Geometry: final body of the model. Coordinates: model frame, mm. Coordinates: 2 decimals unless noted, no trailing zeros. Order: outer loops, then holes, each group sorted by start corner. A loop starts at its lowest first (then second) coordinate and runs counter-clockwise, first axis right, second up. Notation, with made-up numbers: M -7.75,5 L 35.25,5 A8 ccw 35.25,10 Z; hole C 51,-8.75 d2. An arc over 180 degrees is marked long. Use CSV: the item, a comma, the result in double quotes. Start each with the question number.
Q1. Section query A-A, the plane x = 0. Output: boundary loops of the cut face in (y, z), and give its area (3 significant figures).
Q2. Section query B-B, the plane x = -15.5. Output: boundary loops of the cut face in (y, z), and give its area (3 significant figures).
Q3. Ray query, probe 1 along Y at (x, z) = (-15.5, -0.3); probe 2 along X at (y, z) = (-16.5, 0.65); probe 3 along Y at (x, z) = (16, -0.85). Return the intervals inside material, ascending.
Q4. Mould query, pull axis Y, two halves, no side actions, for faces 1 (the face through (-17, 15.57, 0.02)), 2 (the face through (4, 7, 1.5)), 3 (the face through (-2.49, -11.03, 0.02)), 4 (the face through (4, -22.5, 0)). Classes: +Y half, -Y half, draft (parallel to the pull), parting line (faces both ways), or undercut.
Q5. Section query D-D, the plane z = -0.55. State how many separate pieces and enclosed holes the cut face has, and give its area (3 significant figures).
Q6. Section query C-C, the plane y = 15.5. Output: boundary loops of the cut face in (x, z).
Q7. First-contact query: P1, Ø2.5, axis at x = 16.28, y = 19.79, coming from the -Z side. Flat tip, straight axial feed; report the tip coordinate or a pass-through.
from build123d import *

# Parameters (mm, degrees)
SKETCH1_W           = 45
SKETCH1_H           = 45
SKETCH1_R           = 6
BOSS_EXTRUDE1_DEPTH = 1.5
SKETCH4_W           = 3
SKETCH4_H           = 45
BOSS_EXTRUDE2_DEPTH = 20
SKETCH2_R           = 1.5
CUT_EXTRUDE1_DEPTH  = 5
SKETCH3_R           = 1.5
CUT_EXTRUDE2_DEPTH  = 5
SKETCH5_W           = 65
SKETCH5_H           = 3
BOSS_EXTRUDE3_DEPTH = 4.29
SKETCH6_W           = 10.715390309
SKETCH6_H           = 49.29
CUT_EXTRUDE3_DEPTH  = 4.29


with BuildPart() as part:
    # Sketch1 → Boss-Extrude1 (new, symmetric)
    with BuildSketch(Plane.XY):
        Rectangle(SKETCH1_W, SKETCH1_H)
        Circle(SKETCH1_R, mode=Mode.SUBTRACT)
    extrude(amount=BOSS_EXTRUDE1_DEPTH, both=True)

    # Sketch4 → Boss-Extrude2 (add)
    with BuildSketch(Plane(origin=(22.5, 0, 0), x_dir=(0, 0, -1), z_dir=(1, 0, 0))):
        Rectangle(SKETCH4_W, SKETCH4_H)
    extrude(amount=BOSS_EXTRUDE2_DEPTH)

    # Sketch2 → Cut-Extrude1 (cut, symmetric)
    with BuildSketch(Plane.XY.offset(1.5)):
        with Locations((-15.5, 15.5)):
            Circle(SKETCH2_R)
        with Locations((15.5, 15.5)):
            Circle(SKETCH2_R)
        with Locations((15.5, -15.5)):
            Circle(SKETCH2_R)
        with Locations((-15.5, -15.5)):
            Circle(SKETCH2_R)
    extrude(amount=CUT_EXTRUDE1_DEPTH, both=True, mode=Mode.SUBTRACT)

    # Sketch3 → Cut-Extrude2 (cut, symmetric)
    with BuildSketch(Plane.XY.offset(1.5)):
        with Locations((-3.294228634, -12.294228634)):
            Circle(SKETCH3_R)
        with Locations((25.284609691, 4.205771366)):
            Circle(SKETCH3_R)
        with Locations((16.284609691, 19.794228634)):
            Circle(SKETCH3_R)
        with Locations((-12.294228634, 3.294228634)):
            Circle(SKETCH3_R)
    extrude(amount=CUT_EXTRUDE2_DEPTH, both=True, mode=Mode.SUBTRACT)

    # Sketch5 → Boss-Extrude3 (add)
    with BuildSketch(Plane(origin=(0, 22.5, 0), x_dir=(1, 0, 0), z_dir=(0, 1, 0))):
        with Locations((10, 0)):
            Rectangle(SKETCH5_W, SKETCH5_H)
    extrude(amount=BOSS_EXTRUDE3_DEPTH)

    # Sketch6 → Cut-Extrude3 (cut)
    with BuildSketch(Plane.XY.offset(1.5)):
        with Locations((37.142304845, 2.145)):
            Rectangle(SKETCH6_W, SKETCH6_H)
    extrude(amount=-CUT_EXTRUDE3_DEPTH, mode=Mode.SUBTRACT)


solid = part.part
Responses:
1,outline,"M -22.5,-1.5 L -6,-1.5 L -6,1.5 L -22.5,1.5 Z; M 6,-1.5 L 26.79,-1.5 L 26.79,1.5 L 6,1.5 Z"
1,area,"112 mm²"
2,outline,"M -22.5,-1.5 L -17,-1.5 L -17,1.5 L -22.5,1.5 Z; M -14,-1.5 L 14,-1.5 L 14,1.5 L -14,1.5 Z; M 17,-1.5 L 26.79,-1.5 L 26.79,1.5 L 17,1.5 Z"
2,area,"130 mm²"
3,probe 1,"y = -22.5 to -17, -14 to 14, 17 to 26.79"
3,probe 2,"x = -22.5 to -16.62, -14.38 to 14.38, 16.62 to 31.78"
3,probe 3,"y = -22.5 to -16.91, -14.09 to 14.09, 16.91 to 18.32, 21.27 to 26.79"
4,face 1,"undercut"
4,face 2,"draft"
4,face 3,"undercut"
4,face 4,"-Y half"
5,separate pieces,"1"
5,enclosed holes,"9"
5,area,"2,510 mm²"
6,outline,"M -22.5,-1.5 L -17,-1.5 L -17,1.5 L -22.5,1.5 Z; M -14,-1.5 L 14,-1.5 L 14,1.5 L -14,1.5 Z; M 17,-1.5 L 31.78,-1.5 L 31.78,1.5 L 17,1.5 Z"
7,P1,"passes through"
